```python
from build123d import *

# Parameters (mm, degrees)
SKETCH_1_R          = 33.5
SKETCH_1_R_2        = 25
SKETCH_1_W          = 80
SKETCH_1_H          = 20
SKETCH_1_R_3        = 2.1
EXTRUDE_1_DEPTH     = 6
SKETCH_3_R          = 2.05
CUT_EXTRUDE_1_DEPTH = 126.686116974
EXTRUDE_2_DEPTH     = 6
FILLET_1_R          = 2
SKETCH_5_W          = 80
SKETCH_5_H          = 3
EXTRUDE_3_DEPTH     = 6
FILLET_2_R          = 5
SKETCH_6_W          = 50
SKETCH_6_H          = 20
CUT_EXTRUDE_2_DEPTH = 10
FILLET_3_R          = 3
FILLET_4_R          = 1.5
FILLET_5_R          = 5


with BuildPart() as part:
    # 草图1 → 凸台-拉伸1 (new body)
    # profile 1 of 3: a face of its own
    with BuildSketch(Plane.XY):
        with Locations((0, 85.5)):
            Circle(SKETCH_1_R)
        with Locations((0, 85.5)):
            Circle(SKETCH_1_R_2, mode=Mode.SUBTRACT)
    # profile 2 of 3: a face of its own
    with BuildSketch(Plane.XY):
        with BuildLine():
            Line((-33.38100662, 88.32106311), (-40, 10))
            Line((-40, 10), (40, 10))
            Line((40, 10), (33.38100662, 88.32106311))
            ThreePointArc((33.38100662, 88.32106311), (33.470238435, 86.911785792), (33.5, 85.5))
            ThreePointArc((33.5, 85.5), (-1.411785792, 52.029761565), (-33.38100662, 88.32106311))
        make_face()
    # profile 3 of 3: a face of its own
    with BuildSketch(Plane.XY):
        Rectangle(SKETCH_1_W, SKETCH_1_H)
        with Locations((-30, 7.5)):
            Circle(SKETCH_1_R_3, mode=Mode.SUBTRACT)
        with Locations((30, 7.5)):
            Circle(SKETCH_1_R_3, mode=Mode.SUBTRACT)
        with Locations((30, -7.5)):
            Circle(SKETCH_1_R_3, mode=Mode.SUBTRACT)
        with Locations((-30, -7.5)):
            Circle(SKETCH_1_R_3, mode=Mode.SUBTRACT)
    extrude(amount=EXTRUDE_1_DEPTH)

    # 草图3 → 切除-拉伸1 (cut, through all)
    with BuildSketch(Plane.XY.offset(6)):
        with Locations((0, 114.5)):
            Circle(SKETCH_3_R)
        with Locations((14.5, 110.61473671)):
            Circle(SKETCH_3_R)
        with Locations((25.11473671, 100)):
            Circle(SKETCH_3_R)
        with Locations((29, 85.5)):
            Circle(SKETCH_3_R)
        with Locations((25.11473671, 71)):
            Circle(SKETCH_3_R)
        with Locations((14.5, 60.38526329)):
            Circle(SKETCH_3_R)
        with Locations((0, 56.5)):
            Circle(SKETCH_3_R)
        with Locations((-14.5, 60.38526329)):
            Circle(SKETCH_3_R)
        with Locations((-25.11473671, 71)):
            Circle(SKETCH_3_R)
        with Locations((-29, 85.5)):
            Circle(SKETCH_3_R)
        with Locations((-25.11473671, 100)):
            Circle(SKETCH_3_R)
        with Locations((-14.5, 110.61473671)):
            Circle(SKETCH_3_R)
    extrude(amount=-CUT_EXTRUDE_1_DEPTH, mode=Mode.SUBTRACT)


with BuildPart() as body_2:
    # 草图4 → 凸台-拉伸2 (new body)
    with BuildSketch(Plane.XY.offset(6)):
        with BuildLine():
            ThreePointArc((-10.272279454, 108.292109925), (-12.5, 107.150635095), (-14.602406473, 105.792109925))
            Line((-14.602406473, 105.792109925), (-9.560163238, 97.058688457))
            Line((-9.560163238, 97.058688457), (-7.77754959, 93.971111048))
            ThreePointArc((-7.77754959, 93.971111048), (-5.75, 95.459292144), (-3.447422571, 96.471111048))
            Line((-3.447422571, 96.471111048), (-5.230036219, 99.558688457))
            Line((-5.230036219, 99.558688457), (-10.272279454, 108.292109925))
        make_face()
        with BuildLine():
            ThreePointArc((25, 85.5), (24.968651828, 86.751569376), (24.874685928, 88))
            Line((24.874685928, 88), (14.790199458, 88))
            Line((14.790199458, 88), (11.22497216, 88))
            ThreePointArc((11.22497216, 88), (11.431036258, 86.757541283), (11.5, 85.5))
            ThreePointArc((11.5, 85.5), (11.431036258, 84.242458717), (11.22497216, 83))
            Line((11.22497216, 83), (14.790199458, 83))
            Line((14.790199458, 83), (24.874685928, 83))
            ThreePointArc((24.874685928, 83), (24.968651828, 84.248430624), (25, 85.5))
        make_face()
        with BuildLine():
            Line((-9.560163238, 73.941311543), (-14.602406473, 65.207890075))
            ThreePointArc((-14.602406473, 65.207890075), (-12.5, 63.849364905), (-10.272279454, 62.707890075))
            Line((-10.272279454, 62.707890075), (-5.230036219, 71.441311543))
            Line((-5.230036219, 71.441311543), (-3.447422571, 74.528888952))
            ThreePointArc((-3.447422571, 74.528888952), (-5.75, 75.540707856), (-7.77754959, 77.028888952))
            Line((-7.77754959, 77.028888952), (-9.560163238, 73.941311543))
        make_face()
        with BuildLine():
            Line((-7.77754959, 93.971111048), (-9.560163238, 97.058688457))
            ThreePointArc((-9.560163238, 97.058688457), (-15, 85.5), (-9.560163238, 73.941311543))
            Line((-9.560163238, 73.941311543), (-7.77754959, 77.028888952))
            ThreePointArc((-7.77754959, 77.028888952), (-11.5, 85.5), (-7.77754959, 93.971111048))
        make_face()
        with BuildLine():
            Line((-3.447422571, 74.528888952), (-5.230036219, 71.441311543))
            ThreePointArc((-5.230036219, 71.441311543), (7.5, 72.509618943), (14.790199458, 83))
            Line((14.790199458, 83), (11.22497216, 83))
            ThreePointArc((11.22497216, 83), (5.75, 75.540707856), (-3.447422571, 74.528888952))
        make_face()
        with BuildLine():
            ThreePointArc((14.790199458, 88), (7.5, 98.490381057), (-5.230036219, 99.558688457))
            Line((-5.230036219, 99.558688457), (-3.447422571, 96.471111048))
            ThreePointArc((-3.447422571, 96.471111048), (5.75, 95.459292144), (11.22497216, 88))
            Line((11.22497216, 88), (14.790199458, 88))
        make_face()
    extrude(amount=-EXTRUDE_2_DEPTH)

    # Combine 1: union part
    add(part.part)

    # 圆角1
    fillet_1_edges = [body_2.edges().sort_by_distance(p)[0] for p in [
        (-9.560163238, 73.941311543, 3),
        (-14.602406473, 65.207890075, 3),
        (-10.272279454, 62.707890075, 3),
        (-5.230036219, 71.441311543, 3),
        (14.790199458, 83, 3),
        (24.874685928, 83, 3),
        (24.874685928, 88, 3),
        (14.790199458, 88, 3),
        (-5.230036219, 99.558688457, 3),
        (-10.272279454, 108.292109925, 3),
        (-14.602406473, 105.792109925, 3),
        (-9.560163238, 97.058688457, 3),
    ]]
    fillet(fillet_1_edges, radius=FILLET_1_R)

    # 草图5 → 凸台-拉伸3 (add)
    with BuildSketch(Plane.XY.offset(6)):
        with Locations((0, -11.5)):
            Rectangle(SKETCH_5_W, SKETCH_5_H)
    extrude(amount=-EXTRUDE_3_DEPTH)

    # 圆角2
    fillet_2_edges = [body_2.edges().sort_by_distance(p)[0] for p in [
        (-40, -13, 3),
        (40, -13, 3),
    ]]
    fillet(fillet_2_edges, radius=FILLET_2_R)

    # 草图6 → 切除-拉伸2 (cut)
    with BuildSketch(Plane(origin=(0, 0, 0), x_dir=(-1, 0, 0), z_dir=(0, 0, -1))):
        with Locations((0, 2)):
            Rectangle(SKETCH_6_W, SKETCH_6_H)
        Polygon((-33.302523575, 18), (-20.950767875, 18), (-30.401818232, 52.323395297), align=None)
        with BuildLine():
            Line((-16.167580049, 26.996929919), (-3.922674029, 48.205729281))
            ThreePointArc((-3.922674029, 48.205729281), (-14.860033774, 51.069934705), (-24.446601804, 57.063866996))
            Line((-24.446601804, 57.063866996), (-16.167580049, 26.996929919))
        make_face()
        with BuildLine():
            ThreePointArc((24.446601804, 57.063866996), (14.860033774, 51.069934705), (3.922674029, 48.205729281))
            Line((3.922674029, 48.205729281), (16.167580049, 26.996929919))
            Line((16.167580049, 26.996929919), (24.446601804, 57.063866996))
        make_face()
        Polygon((30.401818232, 52.323395297), (20.950767875, 18), (33.302523575, 18), align=None)
        Polygon((-13.279056191, 18), (-3, 18), (-3, 35.803847577), align=None)
        Polygon((3, 35.803847577), (3, 18), (13.279056191, 18), align=None)
    extrude(amount=-CUT_EXTRUDE_2_DEPTH, mode=Mode.SUBTRACT)

    # 圆角3
    fillet_3_edges = [body_2.edges().sort_by_distance(p)[0] for p in [
        (-25, 12, 3),
        (-25, -8, 3),
        (25, -8, 3),
        (25, 12, 3),
    ]]
    fillet(fillet_3_edges, radius=FILLET_3_R)

    # 圆角4
    fillet_4_edges = [body_2.edges().sort_by_distance(p)[0] for p in [
        (-3, 35.803847577, 3),
        (-13.279056191, 18, 3),
        (-3, 18, 3),
        (3, 35.803847577, 3),
        (3, 18, 3),
        (13.279056191, 18, 3),
        (-24.446601804, 57.063866996, 3),
        (-16.167580049, 26.996929919, 3),
        (-20.950767875, 18, 3),
        (-30.401818232, 52.323395297, 3),
        (-33.302523575, 18, 3),
        (20.950767875, 18, 3),
        (33.302523575, 18, 3),
        (30.401818232, 52.323395297, 3),
        (24.446601804, 57.063866996, 3),
        (16.167580049, 26.996929919, 3),
    ]]
    fillet(fillet_4_edges, radius=FILLET_4_R)

    # 圆角5
    fillet_5_edges = [body_2.edges().sort_by_distance(p)[0] for p in [
        (-3.922674029, 48.205729281, 3),
        (3.922674029, 48.205729281, 3),
    ]]
    fillet(fillet_5_edges, radius=FILLET_5_R)


solid = body_2.part
```
Part model, mm, in its own coordinate system. A direction names the side the tool comes from. Coordinates: 2 decimals unless noted, no trailing zeros. Order: outer loops, then holes, each group sorted by start corner. A loop starts at its lowest first (then second) coordinate and runs counter-clockwise, first axis right, second up. Notation, with made-up numbers: (74.25, -6) -> (102.25, -6) arc R20 ccw to (102.25, 5) -> close; hole circle Ø2 at (84, 32). An arc over 180 degrees is marked (long way). Put each result on its own line as item: value. Start each with the question number.
(1) Probe line 1 along Y through (x, z) = (-30, 4.7); line 2 along X through (y, z) = (90, 0.5); line 3 along X through (y, z) = (20, 1.5). List the from-to ranges inside material, lowest first. Write a range as [from, to].
(2) Which spindle directions (+Z, -Z, +X, -X, +Y, -Y) get a long thin tool onto all of the face, cutting with end or side? Do faces 5 (the face through (3, 25, 3)), 6 (the face through (-40, 1, 3)). Say none if no direction does.
(3) Pin check, flat tips, straight feed: pin 1 Ø3 at (y, z) = (22.5, 4.5) entering from +X; pin 2 Ø3 at (x, z) = (13, 1) entering from +Y; pin 3 Ø3 at (x, z) = (30, 3) entering from +Y. Stop position of each tip, or through.
(4) Band-saw the part on A-A (y = 114.5). Give the cut face in (x, z).
(5) Mould opens along X. For faces 1 (the face through (36.737, 48.612, 2.958)), 2 (the face through (-36.644, 49.709, 2.958)), 3 (the face through (24.774, 31.886, 2.958)), 4 (the face through (-9.243, 108.012, 2.958)) say: pulls with the +X half, pulls with the -X half, needs draft (parallel to the pull), parting line crosses it, or undercut.
(6) Band-saw the part on B-B (x = 18.5). Give the cut face in (y, z).
(7) Band-saw the part on C-C (z = 2). Count the separate pieces of the cut face and the enclosed holes in it, then the cut area to 3 significant figures.
Determined:
1. line 1: y = [-13, -9.6], [-5.4, 5.4], [9.6, 18], [45.27, 83.71], [87.29, 100.41]
1. line 2: x = [-33.2, -24.59], [-14.31, -10.58], [10.58, 14.31], [24.56, 33.2]
1. line 3: x = [-39.15, -33.13], [-21.5, -12.1], [-3, 3], [12.1, 21.5], [33.13, 39.15]
2. face 5: +Z, -Z
2. face 6: +Z, -Z, -X, +Y, -Y
3. pin 1: stops at x = 39.07
3. pin 2: stops at y = 116.96
3. pin 3: stops at y = 103.11
4. outline: (-16.77, 0) -> (-2.05, 0) -> (-2.05, 6) -> (-16.77, 6) -> close; (2.05, 0) -> (16.77, 0) -> (16.77, 6) -> (2.05, 6) -> close
5. face 1: pulls with the +X half
5. face 2: pulls with the -X half
5. face 3: undercut
5. face 4: undercut
6. outline: (-13, 0) -> (-8, 0) -> (-8, 6) -> (-13, 6) -> close; (12, 0) -> (35.47, 0) -> (35.47, 6) -> (12, 6) -> close; (52.88, 0) -> (68.68, 0) -> (68.68, 6) -> (52.88, 6) -> close; (83, 0) -> (88, 0) -> (88, 6) -> (83, 6) -> close; (102.32, 0) -> (113.43, 0) -> (113.43, 6) -> (102.32, 6) -> close
7. separate pieces: 1
7. enclosed holes: 27
7. area: 5,400 mm²
